CAD build for the part. Positions are in the model's coordinates, mm. Round coordinates to 2 decimals unless told otherwise and drop trailing zeros. Loops run counter-clockwise (first coordinate to the right, second up) from the corner with the lowest first, then second, coordinate; pieces in that order, holes last.
```python
from build123d import *

# Parameters (mm, degrees)
SKETCH1_R           = 2
BOSS_EXTRUDE1_DEPTH = 4
BOSS_EXTRUDE2_START = -4
BOSS_EXTRUDE2_DEPTH = 4
SKETCH3_R           = 1
CUT_EXTRUDE1_DEPTH  = 6.385164807
SKETCH7_R           = 1
BOSS_EXTRUDE4_DEPTH = 2


with BuildPart() as part:
    # Sketch1 → Boss-Extrude1 (new body)
    with BuildSketch(Plane.XY):
        Circle(SKETCH1_R)
    extrude(amount=BOSS_EXTRUDE1_DEPTH)

    # Sketch2 → Boss-Extrude2 (add)
    with BuildSketch(Plane.XY.offset(4).offset(BOSS_EXTRUDE2_START)):
        with BuildLine():
            Line((3, 2), (0, 2))
            ThreePointArc((0, 2), (1.414213562, 1.414213562), (2, 0))
            ThreePointArc((2, 0), (1.414213562, -1.414213562), (0, -2))
            Line((0, -2), (3, -2))
            Line((3, -2), (3, 2))
        make_face()
    extrude(amount=BOSS_EXTRUDE2_DEPTH)

    # Sketch3 → Cut-Extrude1 (cut, through all)
    with BuildSketch(Plane.XY.offset(4)):
        Circle(SKETCH3_R)
    extrude(amount=-CUT_EXTRUDE1_DEPTH, mode=Mode.SUBTRACT)

    # Sketch7 → Boss-Extrude4 (add, symmetric)
    with BuildSketch(Plane(origin=(0, 0, 0), x_dir=(1, 0, 0), z_dir=(0, 1, 0))):
        with BuildLine():
            Line((3, 0), (3, -4))
            Line((3, -4), (6, -4))
            ThreePointArc((6, -4), (8, -2), (6, 0))
            Line((6, 0), (3, 0))
        make_face()
        with Locations(Location((6, -2, 0), (0, 0, 270))):
            Circle(SKETCH7_R, mode=Mode.SUBTRACT)
    extrude(amount=BOSS_EXTRUDE4_DEPTH, both=True)


solid = part.part
```
Item 1: Probe line 1 (X direction, y = -0.2, z = 2.4); line 2 (X direction, y = 0.85, z = 2.1); line 3 (Z direction, x = 6.5, y = 1.2). List the from-to ranges inside material, lowest first.
Answers follow:
line 1: x = -1.99 to -0.98, 0.98 to 5.08, 6.92 to 7.96
line 2: x = -1.81 to -0.53, 0.53 to 5.01, 6.99 to 8
line 3: z = 0.06 to 1.13, 2.87 to 3.94
Item 2: Cut at D-D, the plane y = -1.4. Give the cut face in (x, z).
Answers follow:
outline: (-1.43, 0) - (6, 0) arc R2 ccw to (6, 4) - (-1.43, 4) - close; hole circle Ø2 at (6, 2)
Item 3: Cut at C-C, the plane x = 5.75. Give the cut face in (y, z), plus the area to 3 significant figures.
Answers follow:
outline: (-2, 0) - (2, 0) - (2, 1.03) - (-2, 1.03) - close; (-2, 2.97) - (2, 2.97) - (2, 4) - (-2, 4) - close
area: 8.25 mm2
Item 4: Two-plate mould, pull along Z, no slides. Class faces 1 (the cylindrical face through (7, 0, 2)), 2 (the flat face through (2, 0, 0)), 3 (the flat face through (3, 0, 4)): released by +Z, released by -Z, zero draft, split by the parting line, or undercut.
Answers follow:
face 1: undercut
face 2: released by -Z
face 3: released by +Z
Item 5: Cut at B-B, the plane y = 0. Give the cut face in (x, z), plus the area to 3 significant figures.
Answers follow:
outline: (-2, 0) - (-1, 0) - (-1, 4) - (-2, 4) - close; (1, 0) - (6, 0) arc R2 ccw to (6, 4) - (1, 4) - close; hole circle Ø2 at (6, 2)
area: 27.1 mm2
Item 6: Cut at A-A, the plane z = 2. Give the cut face in (x, y), plus the area to 3 significant figures.
Answers follow:
outline: (0, -2) - (5, -2) - (5, 2) - (0, 2) arc R2 ccw to start; (7, -2) - (8, -2) - (8, 2) - (7, 2) - close; hole circle Ø2 at (0, 0)
area: 27.1 mm2
